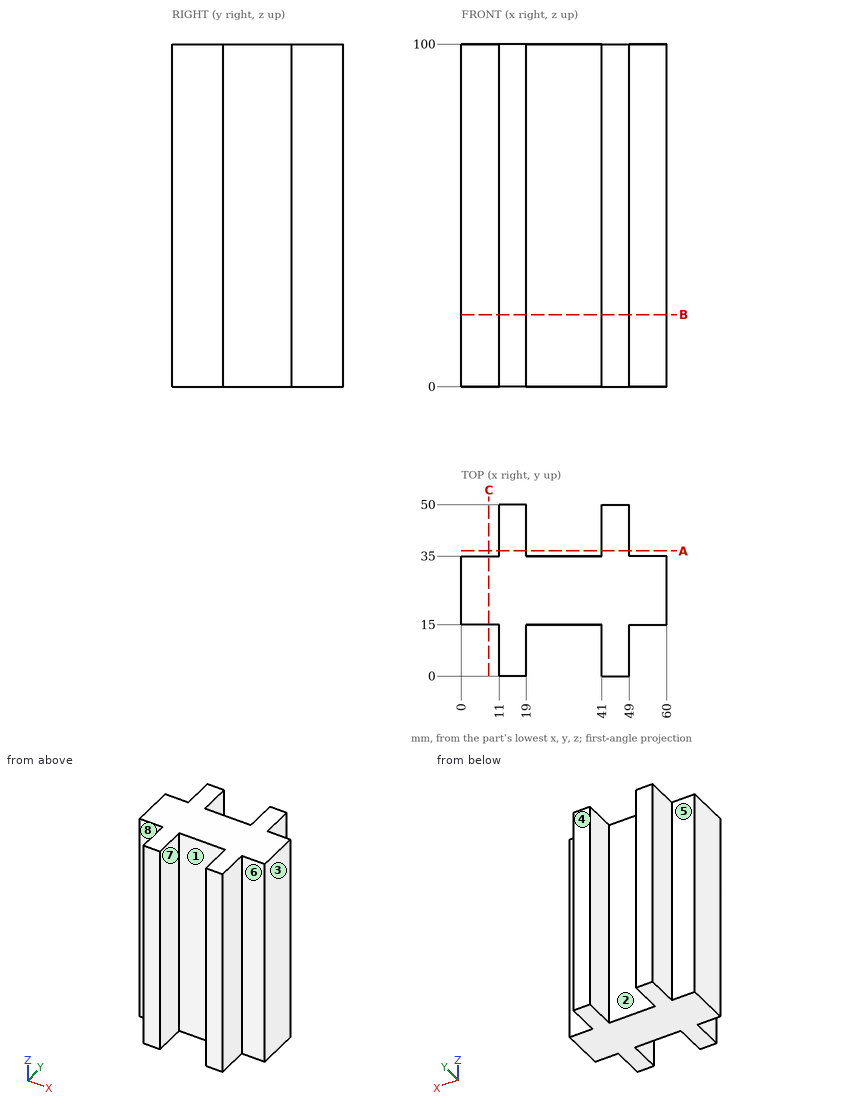
Print and shaded views of the part. All mm, measured from the part's lowest x, y and z. A direction names the side the tool comes from. Round coordinates to 2 decimals unless told otherwise and drop trailing zeros. Write each loop counter-clockwise with the first axis right and the second up, starting at its lowest first coordinate (ties: lowest second). Pieces come first, ordered by that corner, then holes. Notation, with made-up numbers: (36.5, -25) - (88.5, -25) arc R24 cw to (88.5, 0) - close; hole circle Ø2 at (-13, 1). An arc over 180 degrees is marked (long way). Write each question's results on one line, items separated by ' | '. Start each with the question number.
Item 1: Which spindle directions (+Z, -Z, +X, -X, +Y, -Y) get a long thin tool onto all of the face, cutting with end or side? Do the marked faces 5, 6, 7 and 8. Say none if no direction does.
Item 2: Saw through at B-B (z = 21). Write the cut outline in (x, y), and give its area (3 significant figures).
Item 3: Mould opens along X. For the marked faces 1, 2, 3 and 4 say: pulls with the +X half, pulls with the -X half, needs draft (parallel to the pull), parting line crosses it, or undercut.
Item 4: Saw through at C-C (x = 8). Write the cut outline in (y, z).
Item 5: Saw through at A-A (y = 36.5). Write the cut outline in (x, z).
Item 6: Wall check: L1, parallel to X at y = 7.5, z = 58; L2, parallel to Y at x = 54.5, z = 85. Give the ranges that are in metal, low to high. Write a range as [from, to].
Item 7: Drop flat-ended pins along their axis: P1, Ø4, axis at x = 33, z = 86, coming from the +Y side; P2, Ø5.5, axis at x = 4, z = 26.5, coming from the -Y side; P3, Ø12, axis at y = 4, z = 27, coming from the +X side. Give the stop position or say it passes through.
Results are:
1) face 5: +Z, -Z, -X, +Y | face 6: +Z, -Z, +X, -Y | face 7: +Z, -Z, -Y | face 8: +Z, -Z, -X, -Y
2) outline: (0, 15) - (11, 15) - (11, 0) - (19, 0) - (19, 15) - (41, 15) - (41, 0) - (49, 0) - (49, 15) - (60, 15) - (60, 35) - (49, 35) - (49, 50) - (41, 50) - (41, 35) - (19, 35) - (19, 50) - (11, 50) - (11, 35) - (0, 35) - close | area: 1,680 mm²
3) face 1: undercut | face 2: undercut | face 3: pulls with the +X half | face 4: needs draft
4) outline: (15, 0) - (35, 0) - (35, 100) - (15, 100) - close
5) outline: (11, 0) - (19, 0) - (19, 100) - (11, 100) - close; (41, 0) - (49, 0) - (49, 100) - (41, 100) - close
6) L1: x = [11, 19], [41, 49] | L2: y = [15, 35]
7) P1: stops at y = 35 | P2: stops at y = 15 | P3: stops at x = 49
